Build history of the part. All positions in model axes, mm. A direction names the side the tool comes from. Round coordinates to 2 decimals unless told otherwise and drop trailing zeros. Order: outer loops, then holes, each group sorted by start corner. A loop starts at its lowest first (then second) coordinate and runs counter-clockwise, first axis right, second up. Notation, with made-up numbers: (1.25, -7) -> (20.25, -7) arc R19 ccw to (20.25, 17) -> close; hole circle Ø10 at (33.25, -15.5). An arc over 180 degrees is marked (long way). Answer as a JSON object with one key per item and string values.
from build123d import *

# Parameters (mm, degrees)
F0_W      = 1200
F0_H      = 600
F1_DEPTH  = 18
F2_W      = 600
F2_H      = 1200
F3_DEPTH  = 18
F4_W      = 18
F4_H      = 600
F4_W_2    = 600
F4_H_2    = 18
F5_DEPTH  = 732
F6_W      = 18
F6_H      = 1132
F7_DEPTH  = 732
F8_DEPTH  = 18
F9_W      = 1732
F9_H      = 18
F10_DEPTH = 732


with BuildPart() as f1:
    # F0 (on Top) → F1 (new body)
    with BuildSketch(Plane.XY):
        with Locations((600, 300)):
            Rectangle(F0_W, F0_H)
    extrude(amount=F1_DEPTH)

    # F2 (on Top) → F3 (join)
    with BuildSketch(Plane.XY):
        with Locations((-300, 600)):
            Rectangle(F2_W, F2_H)
    extrude(amount=F3_DEPTH)

    # F4 (on face) → F5 (join)
    with BuildSketch(Plane(origin=(0, 0, 0), x_dir=(1, 0, 0), z_dir=(0, 0, -1))):
        with Locations((1141, -300)):
            Rectangle(F4_W, F4_H)
        with Locations((-300, -1141)):
            Rectangle(F4_W_2, F4_H_2)
    extrude(amount=F5_DEPTH)

    # F6 (on face) → F7 (join)
    with BuildSketch(Plane(origin=(0, 0, 0), x_dir=(1, 0, 0), z_dir=(0, 0, -1))):
        with Locations((-409, -566)):
            Rectangle(F6_W, F6_H)
    extrude(amount=F7_DEPTH)

    # F7_face (on face) → F8 (join)
    with BuildSketch(Plane(origin=(259.6, 406.4, 0), x_dir=(1, 0, 0), z_dir=(0, 0, -1))):
        Polygon((872.4, 406.4), (-659.6, 406.4), (-659.6, -725.6), (-259.6, -725.6), (-259.6, -193.6), (872.4, -193.6), align=None)
    extrude(amount=-F8_DEPTH)

    # F9 (on face) → F10 (join)
    with BuildSketch(Plane(origin=(0, 0, 0), x_dir=(1, 0, 0), z_dir=(0, 0, -1))):
        with Locations((266, -191)):
            Rectangle(F9_W, F9_H)
    extrude(amount=F10_DEPTH)


solid = f1.part
1) Which spindle directions (+Z, -Z, +X, -X, +Y, -Y) get a long thin tool onto all of the face, cutting with end or side? Do faces 1 (the face through (-418, 92, -361)), 2 (the face through (1150, 304, -361)), 3 (the face through (-304, 1150, -361)). Say none if no direction does.
Checked values:
{"face 1": "-Z, -X, -Y", "face 2": "-Z, +X, +Y, -Y", "face 3": "-Z, +X, -X, +Y"}
2) Cut at A-A, the plane x = -251. Give the cut face in (y, z).
Checked values:
{"outline": "(0, 0) -> (182, 0) -> (182, -732) -> (200, -732) -> (200, 0) -> (1132, 0) -> (1132, -732) -> (1150, -732) -> (1150, 0) -> (1200, 0) -> (1200, 18) -> (0, 18) -> close"}
3) Cut at C-C, the plane z = -171.5. Give the cut face in (x, y), plus the area to 3 significant figures.
Checked values:
{"outline": "(-600, 182) -> (-418, 182) -> (-418, 0) -> (-400, 0) -> (-400, 182) -> (1132, 182) -> (1132, 0) -> (1150, 0) -> (1150, 600) -> (1132, 600) -> (1132, 200) -> (-400, 200) -> (-400, 1132) -> (0, 1132) -> (0, 1150) -> (-600, 1150) -> (-600, 1132) -> (-418, 1132) -> (-418, 200) -> (-600, 200) -> close", "area": "72,800 mm²"}
4) Cut at D-D, the plane x = 815.5. Give the cut face in (y, z).
Checked values:
{"outline": "(0, 0) -> (182, 0) -> (182, -732) -> (200, -732) -> (200, 0) -> (600, 0) -> (600, 18) -> (0, 18) -> close"}
5) Cut at B-B, the plane y = 681. Give the cut face in (x, z), plus the area to 3 significant figures.
Checked values:
{"outline": "(-600, 0) -> (-418, 0) -> (-418, -732) -> (-400, -732) -> (-400, 0) -> (0, 0) -> (0, 18) -> (-600, 18) -> close", "area": "24,000 mm²"}
6) Flat gauge pins, fed straight in: pin 1 Ø3 at (x, z) = (-340.5, -511.5) entering from +Y; pin 2 Ø3 at (y, z) = (532, -290.5) entering from -X; pin 3 Ø4 at (x, y) = (-386, 951.5) entering from -Z. Where does each tip first touch, or does it go through?
Checked values:
{"pin 1": "stops at y = 1150", "pin 2": "stops at x = -418", "pin 3": "stops at z = 0"}
7) Pull direction Y, two halves, no side cores. Call faces 4 (the face through (1175, 304, 0)), 5 (the face through (355, 182, -361)), 6 (the face through (597, 600, 2)), 7 (the face through (-203, 1132, -361)): pulls with the +Y half, pulls with the -Y half, needs draft (parallel to the pull), parting line crosses it, or undercut.
Checked values:
{"face 4": "needs draft", "face 5": "pulls with the -Y half", "face 6": "pulls with the +Y half", "face 7": "undercut"}
8) Probe L1, parallel to X at y = 392, z = -358; L2, parallel to Y at x = -68, z = -477.5; L3, parallel to Z at x = -67, y = 607. List the from-to ranges inside material, lowest first. Write a range as from..to.
Checked values:
{"L1": "x = -418..-400, 1132..1150", "L2": "y = 182..200, 1132..1150", "L3": "z = 0..18"}
